from build123d import *

# Parameters (mm, degrees)
SKETCH1_R           = 40
SKETCH1_R_2         = 35
BOSS_EXTRUDE1_DEPTH = 10


with BuildPart() as part:
    # Sketch1 → Boss-Extrude1 (new body)
    with BuildSketch(Plane(origin=(0, 0, 0), x_dir=(1, 0, 0), z_dir=(0, 1, 0))):
        Circle(SKETCH1_R)
        Circle(SKETCH1_R_2, mode=Mode.SUBTRACT)
        with BuildLine():
            Line((-6, 0), (-6, 6))
            Line((-6, 6), (-34.481879299, 6))
            ThreePointArc((-34.481879299, 6), (-35, 0), (-34.481879299, -6))
            Line((-34.481879299, -6), (-6, -6))
            Line((-6, -6), (-6, 0))
        make_face()
        with BuildLine():
            Line((6, -34.481879299), (6, -6))
            Line((6, -6), (0, -6))
            Line((0, -6), (-6, -6))
            Line((-6, -6), (-6, -34.481879299))
            ThreePointArc((-6, -34.481879299), (0, -35), (6, -34.481879299))
        make_face()
        with BuildLine():
            Line((6, 6), (6, 0))
            Line((6, 0), (6, -6))
            Line((6, -6), (34.481879299, -6))
            ThreePointArc((34.481879299, -6), (34.870229247, -3.011164603), (35, 0))
            ThreePointArc((35, 0), (34.870229247, 3.011164603), (34.481879299, 6))
            Line((34.481879299, 6), (6, 6))
        make_face()
        with BuildLine():
            Line((0, 6), (6, 6))
            Line((6, 6), (6, 34.481879299))
            ThreePointArc((6, 34.481879299), (0, 35), (-6, 34.481879299))
            Line((-6, 34.481879299), (-6, 6))
            Line((-6, 6), (0, 6))
        make_face()
        with BuildLine():
            Line((-6, -6), (0, -6))
            ThreePointArc((0, -6), (-4.242640687, -4.242640687), (-6, 0))
            Line((-6, 0), (-6, -6))
        make_face()
        with BuildLine():
            Line((6, -6), (6, 0))
            ThreePointArc((6, 0), (4.242640687, -4.242640687), (0, -6))
            Line((0, -6), (6, -6))
        make_face()
        with BuildLine():
            ThreePointArc((0, 6), (4.242640687, 4.242640687), (6, 0))
            Line((6, 0), (6, 6))
            Line((6, 6), (0, 6))
        make_face()
        with BuildLine():
            ThreePointArc((-6, 0), (-4.242640687, 4.242640687), (0, 6))
            Line((0, 6), (-6, 6))
            Line((-6, 6), (-6, 0))
        make_face()
    extrude(amount=BOSS_EXTRUDE1_DEPTH)


solid = part.part
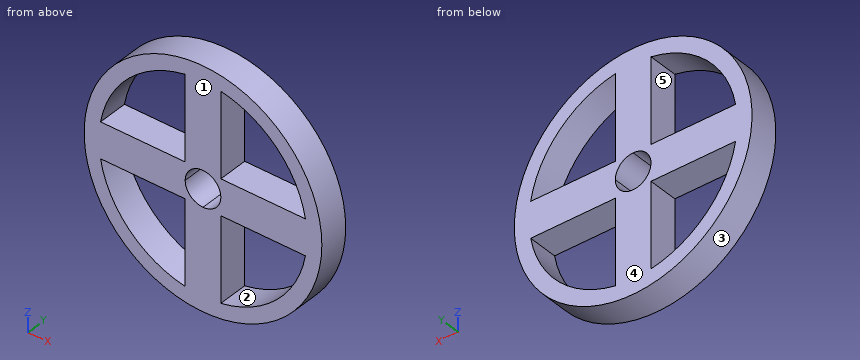
The listing builds one solid part. Answer for the finished solid, in the listing's coordinates (mm). Face numbers are marked on the shaded views. A direction names the side the tool comes from. Round coordinates to 2 decimals unless told otherwise and drop trailing zeros. Write each loop counter-clockwise with the first axis right and the second up, starting at its lowest first coordinate (ties: lowest second). Pieces come first, ordered by that corner, then holes. Notation, with made-up numbers: M 66,31.25 L 73,31.25 A22 cw 73,70.25 Z; hole C 4,68 d3. An arc over 180 degrees is marked long. Write each question's results on one line, items separated by ' | '. Start each with the question number.
(1) The part is cut by section D-D, the plane z = 5. Write down the section's boundary in (x, y), and give its area (3 significant figures).
(2) The part is cut by section A-A, the plane z = 29. Write down the section's boundary in (x, y).
(3) For the marked faces 4 and 5, determine the directions among +Z, -Z, +X, -X, +Y, -Y from which every point of the face is accessible in a straight line to the end or side of a thin tool.
(4) Determine the mould class of the marked faces 1, 2 and 3 for opening direction X: +X half, -X half, draft (parallel to the pull), parting line (faces both ways), or undercut.
(5) Find the intervals of material crossed by line 1 (Z direction, x = -21, y = 4.75); line 2 (X direction, y = 5, z = 30); line 3 (Z direction, x = -6.5, y = 6.75), in increasing order.
(6) Each of these flat-tipped pins is pushed along its axis until it touches: P1, Ø5, axis at x = -19, z = 25, coming from the -Y side; P2, Ø5, axis at x = 22.5, y = 7, coming from the +Z side; P3, Ø5, axis at y = 4, z = 18.5, coming from the -X side; P4, Ø3, axis at y = 6.5, z = -26, coming from the +X side. Where does it stop, or does it pass through?
(7) The part is cut by section C-C, the plane x = 12. Write down the section's boundary in (y, z).
(8) The part is cut by section B-B, the plane y = 6.75. Write down the section's boundary in (x, z).
Worked answers:
1) outline: M -39.69,0 L -3.32,0 L -3.32,10 L -39.69,10 Z; M 3.32,0 L 39.69,0 L 39.69,10 L 3.32,10 Z | area: 727 mm²
2) outline: M -27.55,0 L -19.6,0 L -19.6,10 L -27.55,10 Z; M -6,0 L 6,0 L 6,10 L -6,10 Z; M 19.6,0 L 27.55,0 L 27.55,10 L 19.6,10 Z
3) face 4: +Z, -Z, +X, -X, +Y | face 5: +Y, -Y
4) face 1: draft | face 2: undercut | face 3: parting line
5) line 1: z = -34.04 to -28, -6 to 6, 28 to 34.04 | line 2: x = -26.46 to -18.03, -6 to 6, 18.03 to 26.46 | line 3: z = -39.47 to -34.39, -6 to 6, 34.39 to 39.47
6) P1: passes through | P2: stops at z = 34.64 | P3: stops at x = -36.66 | P4: stops at x = 31.62
7) outline: M 0,-38.16 L 10,-38.16 L 10,-32.88 L 0,-32.88 Z; M 0,-6 L 10,-6 L 10,6 L 0,6 Z; M 0,32.88 L 10,32.88 L 10,38.16 L 0,38.16 Z
8) outline: C 0,0 d80; hole M -34.48,-6 A35 ccw -6,-34.48 L -6,-6 Z; hole M -34.48,6 L -6,6 L -6,34.48 A35 ccw Z; hole C 0,0 d12; hole M 6,-34.48 A35 ccw 34.48,-6 L 6,-6 Z; hole M 6,6 L 34.48,6 A35 ccw 6,34.48 Z
